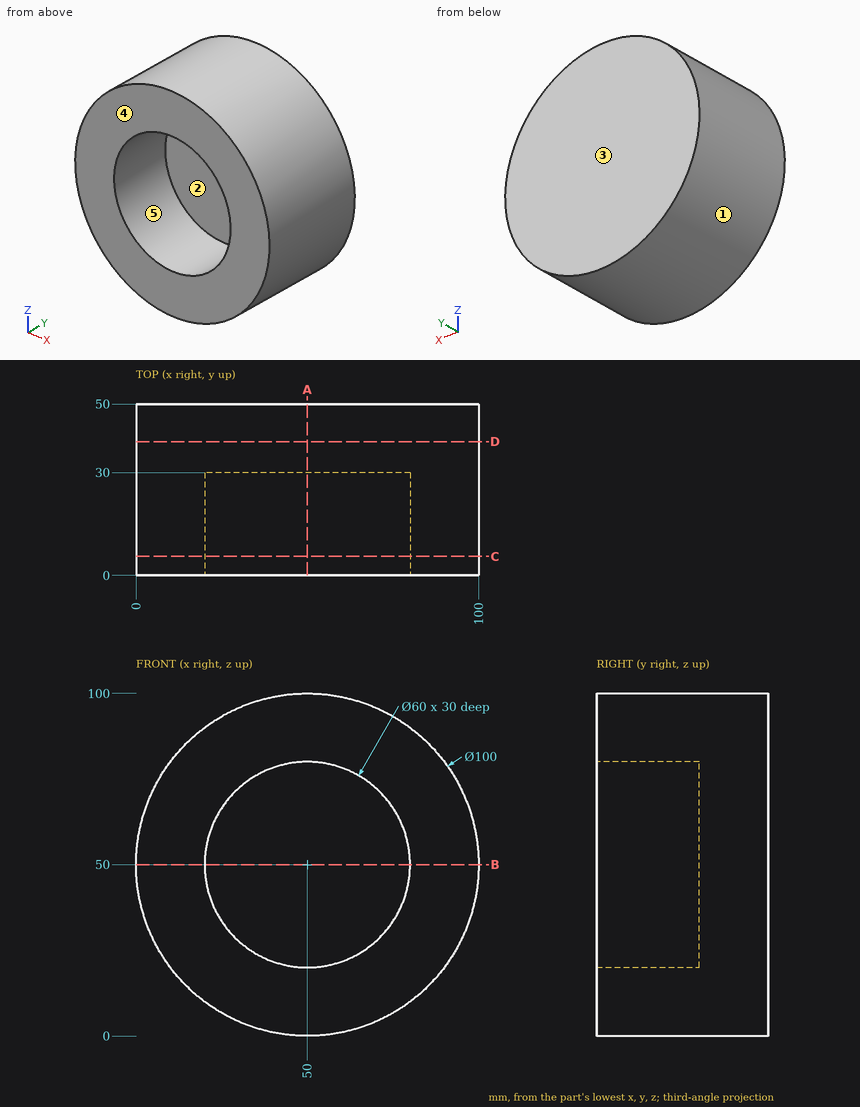
For this review, use the dimensioned drawing (mm, ordinates from the lowest corner) and the shaded views. A direction names the side the tool comes from. Coordinates: 2 decimals unless noted, no trailing zeros. Loops run counter-clockwise (first coordinate to the right, second up) from the corner with the lowest first, then second, coordinate; pieces in that order, holes last. Notation, with made-up numbers: (49.25, 69.25) -> (91.25, 69.25) arc R21 cw to (91.25, 79.25) -> close; hole circle Ø11 at (7, 71.5). An arc over 180 degrees is marked (long way). Use a Markdown table: item, result. Add a question column.
1. Add section A-A on x = 50. Write out the cut boundary in (y, z), plus the area to 3 significant figures.
2. Add section C-C on y = 5.5. Write out the cut boundary in (x, z), plus the area to 3 significant figures.
3. Machinability: for the marked faces 4 and 5, which of the approach directions +Z, -Z, +X, -X, +Y, -Y give a long, thin tool a straight path to every point of the face, cutting with its end or side? Answer none if there is none.
4. Draft analysis for pull direction X (two halves, no side actions). For the marked faces 1, 2 and 3, state which applies: pulls with the +X half, pulls with the -X half, needs draft (parallel to the pull), parting line crosses it, or undercut.
5. To check wall thickness, follow line 1 (X direction, y = 10, z = 50); line 2 (Z direction, x = 51, y = 24.5); line 3 (Y direction, x = 77.5, z = 52). State the ranges of each line that lie inside material, in increasing order.
6. Add section D-D on y = 39. Write out the cut boundary in (x, z), plus the area to 3 significant figures.
7. Clearance check with flat-ended pins moving along their axes: pin 1 Ø8 at (x, y) = (25.5, 31.5) entering from +Z; pin 2 Ø6 at (x, y) = (27.5, 34.5) entering from +Z; pin 3 Ø12 at (x, y) = (26.5, 34.5) entering from +Z. State where each tip first meets the part, or that it passes through.
8. Add section B-B on z = 50. Write out the cut boundary in (x, y).
Returned:
| question | item | result |
|---|---|---|
| 1 | outline | (0, 0) -> (50, 0) -> (50, 100) -> (0, 100) -> (0, 80) -> (30, 80) -> (30, 20) -> (0, 20) -> close |
| 1 | area | 3,200 mm² |
| 2 | outline | circle Ø100 at (50, 50); hole circle Ø60 at (50, 50) |
| 2 | area | 5,030 mm² |
| 3 | face 4 | +Z, -Z, +X, -X, -Y |
| 3 | face 5 | -Y |
| 4 | face 1 | parting line crosses it |
| 4 | face 2 | undercut |
| 4 | face 3 | needs draft |
| 5 | line 1 | x = 0 to 20, 80 to 100 |
| 5 | line 2 | z = 0.01 to 20.02, 79.98 to 99.99 |
| 5 | line 3 | y = 30 to 50 |
| 6 | outline | circle Ø100 at (50, 50) |
| 6 | area | 7,850 mm² |
| 7 | pin 1 | stops at z = 95.6 |
| 7 | pin 2 | stops at z = 96.04 |
| 7 | pin 3 | stops at z = 96.84 |
| 8 | outline | (0, 0) -> (20, 0) -> (20, 30) -> (80, 30) -> (80, 0) -> (100, 0) -> (100, 50) -> (0, 50) -> close |
